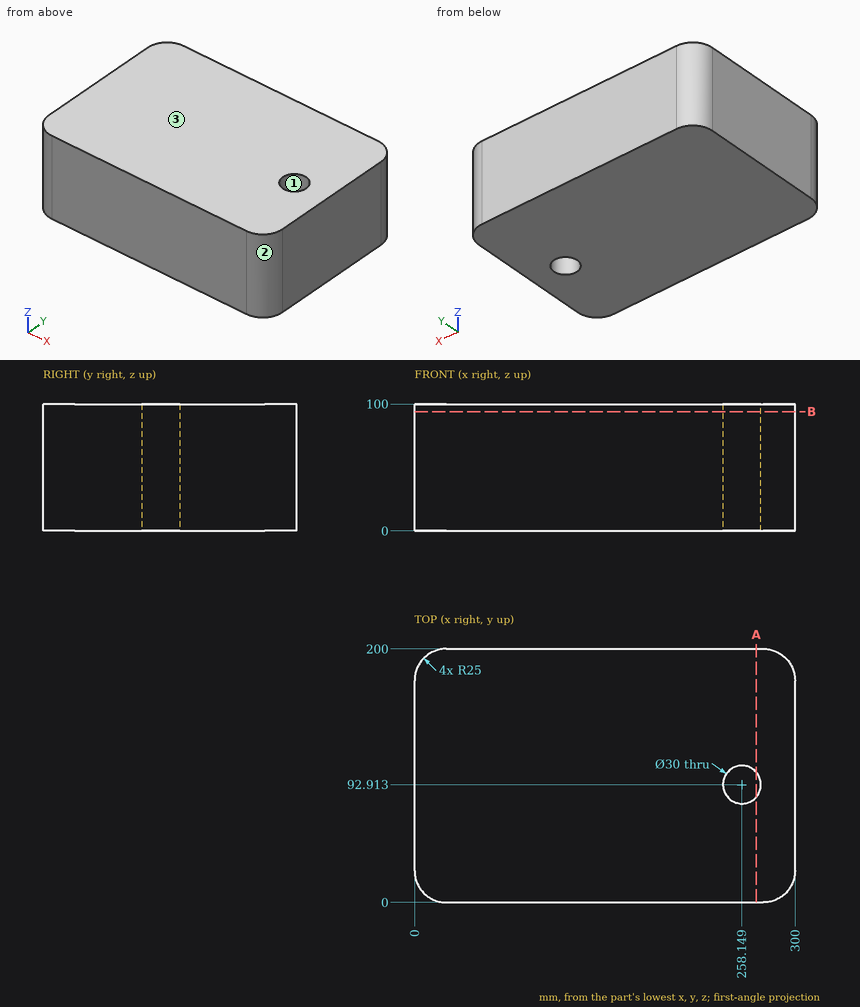
The figure shows three views and two pictorial views of one solid part (mm, origin at its lowest corner). Answer the questions. Coordinates: 2 decimals unless noted, no trailing zeros. Loops run counter-clockwise (first coordinate to the right, second up) from the corner with the lowest first, then second, coordinate; pieces in that order, holes last.
1) Find section A-A on x = 269.5. Write down the section's boundary in (y, z), then the cut area to 3 significant figures.
2) Find the intervals of material crossed by L1, parallel to Y at x = 258, z = 35; L2, parallel to Y at x = 253, z = 45 (1 decimal); L3, parallel to X at y = 12, z = 39.5 (1 decimal), in increasing order.
3) Find section B-B on z = 94. Write down the section's boundary in (x, y).
4) Determine the mould class of the marked faces 1, 2 and 3 for opening direction X: pulls with the +X half, pulls with the -X half, needs draft (parallel to the pull), parting line crosses it, or undercut.
Values:
1. outline: (0, 0) - (83.11, 0) - (83.11, 100) - (0, 100) - close; (102.72, 0) - (200, 0) - (200, 100) - (102.72, 100) - close
1. area: 18,000 mm2
2. L1: y = 0 to 77.91, 107.91 to 200
2. L2: y = 0 to 78.8, 107 to 200
2. L3: x = 3.6 to 296.4
3. outline: (0, 25) arc R25 ccw to (25, 0) - (275, 0) arc R25 ccw to (300, 25) - (300, 175) arc R25 ccw to (275, 200) - (25, 200) arc R25 ccw to (0, 175) - close; hole circle Ø30 at (258.15, 92.91)
4. face 1: undercut
4. face 2: pulls with the +X half
4. face 3: needs draft
